Verification items for this drawing (mm, ordinates from the low corner). A direction names the side the tool comes from. Give positions to 0.01 mm unless a question says otherwise; leave off trailing zeros. Write each loop counter-clockwise with the first axis right and the second up, starting at its lowest first coordinate (ties: lowest second). Pieces come first, ordered by that corner, then holes. Notation, with made-up numbers: (50.25, -31.75) -> (71.25, -31.75) arc R8 cw to (71.25, -18.75) -> close; hole circle Ø1 at (-4, -25). An arc over 180 degrees is marked (long way). Use one line per item in the form item = value. Start each with the question number.
(1) Scan lines: L1, parallel to X at y = 14.25, z = 6.5 (1 decimal); L2, parallel to Y at x = 22, z = 9.5 (1 decimal); L3, parallel to X at y = 6.75, z = 14 (1 decimal). Record each from-to range of solid material in increasing order.
(2) Set-up check for the marked faces 1, 2 and 3: record each of +Z, -Z, +X, -X, +Y, -Y from which the full face is reachable in a straight line by a thin tool's end or side.
(3) Section check C-C, the plane z = 4. Record the cut outline in (x, y) (1 decimal).
(4) Release check for a two-part mould opening along Y. For the marked faces 4, 5, 6 and 7 record: pulls with the +Y half, pulls with the -Y half, needs draft (parallel to the pull), parting line crosses it, or undercut.
(5) Section check B-B, the plane x = 5.08. Record the cut outline in (y, z) (1 decimal).
(6) Section check A-A, the plane y = 9. Record the cut outline in (x, z).
(7) Section check D-D, the plane y = 13. State how many separate pieces and enclosed holes the cut face has, plus the area to 3 significant figures.
(8) Depth check by flat-ended pin: pin 1 Ø7 at (x, y) = (39.5, 18) entering from +Z; pin 2 Ø5 at (y, z) = (23, 13) entering from -X; pin 3 Ø4 at (x, y) = (5.08, 14.605) entering from +Z; pin 4 Ø4.5 at (y, z) = (12, 25) entering from +X. Enter the tip coordinate at first touch or a pass-through.
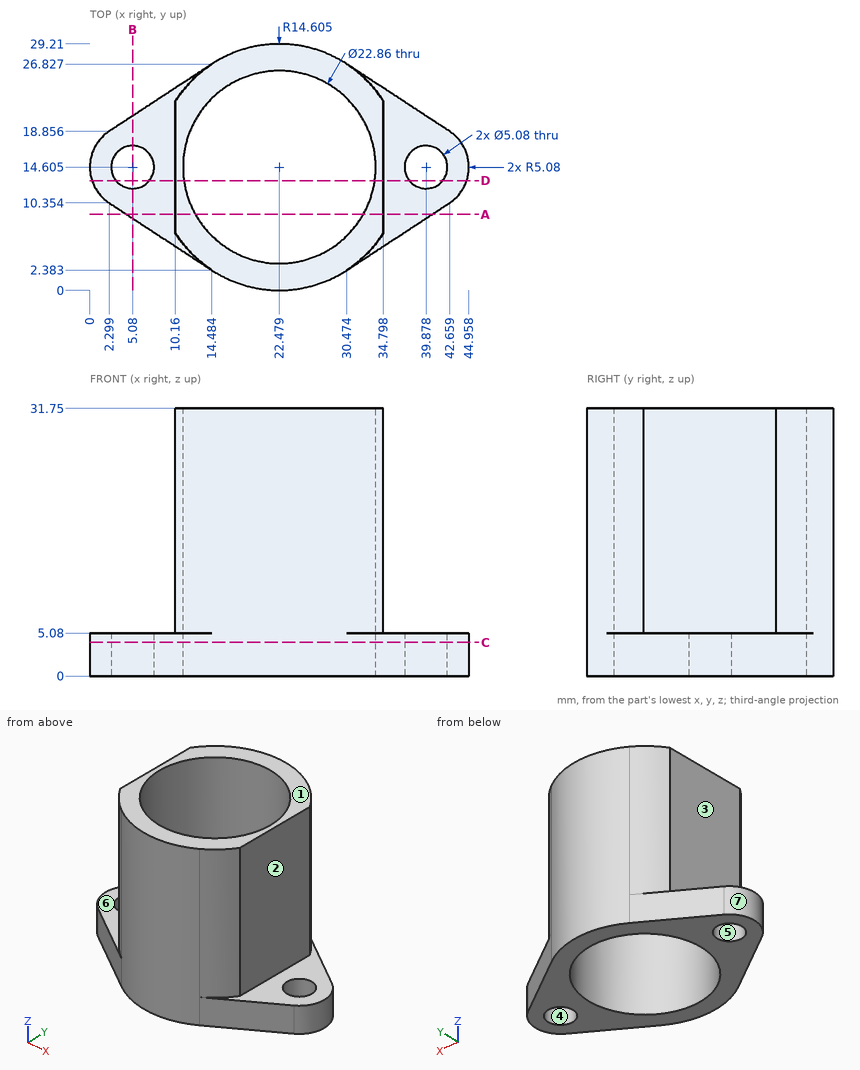
Completed:
q1.L1 = 10.2 to 11.1, 33.9 to 34.8
q1.L2 = 0 to 3.2, 26 to 29.2
q1.L3 = 10.2 to 14.2, 30.8 to 34.8
q2.face_1 = +Z, +X, -X, +Y, -Y
q2.face_2 = +Z, +X, +Y, -Y
q2.face_3 = +Z, -X, +Y, -Y
q3.outline = (2.3, 10.4) -> (14.5, 2.4) arc R14.6 ccw to (30.5, 2.4) -> (42.7, 10.4) arc R5.1 ccw to (42.7, 18.9) -> (30.5, 26.8) arc R14.6 ccw to (14.5, 26.8) -> (2.3, 18.9) arc R5.1 ccw to start; hole circle Ø5.1 at (5.1, 14.6); hole circle Ø22.9 at (22.5, 14.6); hole circle Ø5.1 at (39.9, 14.6)
q4.face_4 = undercut
q4.face_5 = undercut
q4.face_6 = needs draft
q4.face_7 = parting line crosses it
q5.outline = (8.5, 0) -> (12.1, 0) -> (12.1, 5.1) -> (8.5, 5.1) -> close; (17.1, 0) -> (20.7, 0) -> (20.7, 5.1) -> (17.1, 5.1) -> close
q6.outline = (4.37, 0) -> (12.52, 0) -> (12.52, 31.75) -> (10.16, 31.75) -> (10.16, 5.08) -> (4.37, 5.08) -> close; (32.44, 0) -> (40.59, 0) -> (40.59, 5.08) -> (34.8, 5.08) -> (34.8, 31.75) -> (32.44, 31.75) -> close
q7.separate_pieces = 4
q7.enclosed_holes = 0
q7.area = 124 mm²
q8.pin_1 = 5.08
q8.pin_2 = 10.16
q8.pin_3 = through
q8.pin_4 = 34.8
